Autodesk Inventor part; units mm, degrees
ref_plane "YZ Plane" through (0, 0, 0) normal (1, 0, 0) x (0, 1, 0)
ref_plane "XZ Plane" through (0, 0, 0) normal (0, 1, 0) x (-1, 0, 0)
ref_plane "XY Plane" through (0, 0, 0) normal (0, 0, 1) x (1, 0, 0)
sketch "Sketch1" plane through (0, 0, 0) normal (0, 0, 1) x (1, 0, 0)
  line L0 (-8.7146, 7.551) -> (3.2854, 7.551)
  line L1 (3.2854, 7.551) -> (3.2854, 3.051)
  line L2 (3.2854, 3.051) -> (-8.7146, 3.051)
  line L3 (-8.7146, 3.051) -> (-8.7146, 7.551)
  line L4 (2.7854, 7.051) -> (-8.2146, 7.051)
  line L5 (-8.2146, 7.051) -> (-8.2146, 3.551)
  line L6 (-8.2146, 3.551) -> (2.7854, 3.551)
  line L7 (2.7854, 3.551) -> (2.7854, 7.051)
  point P0 (0, 0)
  dimension "d0" = 12
  dimension "d1" = 4.5
  dimension "d2" = 0.5
extrude "Extrusion1" add sketch "Sketch1" along normal blind 15
properties part number "capa" material "Steel, Alloy"
CAD build for the part. Positions are in the model's coordinates, mm. A direction names the side the tool comes from. Round coordinates to 2 decimals unless told otherwise and drop trailing zeros. Write each loop counter-clockwise with the first axis right and the second up, starting at its lowest first coordinate (ties: lowest second). Pieces come first, ordered by that corner, then holes. Notation, with made-up numbers: (4, 28) - (52, 28) arc R32 ccw to (52, 65) - close; hole circle Ø5 at (7.25, -40). An arc over 180 degrees is marked (long way). Write item = value, one per line. Start each with the question number.
Q1. Probe L1, parallel to X at y = 5.65, z = 4.25; L2, parallel to Y at x = -1.5, z = 8.25. List the from-to ranges inside material, lowest first. Write a range as from..to.
Q2. Drop a flat-ended pin along its axis: pin 1 (2 mm diameter, centred on x = -3, y = 5, fed in from -Z). Give the stop position or say it passes through.
Q3. Band-saw the part on B-B (x = -5). Give the cut face in (y, z), then the cut area to 3 significant figures.
Q4. Band-saw the part on C-C (z = 9.25). Give the cut face in (x, y).
Q5. Which spindle directions (+Z, -Z, +X, -X, +Y, -Y) get a long thin tool onto all of the face, cutting with end or side? Do faces 5 (the flat face through (-3, 3.551, 7)), 6 (the flat face through (-3, 7.551, 7)). Say none if no direction does.
Q6. Mould opens along X. For faces 1 (the flat face through (-3, 7.051, 7)), 2 (the flat face through (-8.715, 5, 7)), 3 (the flat face through (-8.215, 5, 7)), 4 (the flat face through (-2.7, 3.3, 15)) say: pulls with the +X half, pulls with the -X half, needs draft (parallel to the pull), parting line crosses it, or undercut.
Q7. Band-saw the part on A-A (y = 5.8). Give the cut face in (x, z).
Answers below:
q1.L1 = -8.71..-8.21, 2.79..3.29
q1.L2 = 3.05..3.55, 7.05..7.55
q2.pin_1 = through
q3.outline = (3.05, 0) - (3.55, 0) - (3.55, 15) - (3.05, 15) - close; (7.05, 0) - (7.55, 0) - (7.55, 15) - (7.05, 15) - close
q3.area = 15.0 mm2
q4.outline = (-8.71, 3.05) - (3.29, 3.05) - (3.29, 7.55) - (-8.71, 7.55) - close; hole (-8.21, 3.55) - (2.79, 3.55) - (2.79, 7.05) - (-8.21, 7.05) - close
q5.face_5 = +Z, -Z
q5.face_6 = +Z, -Z, +X, -X, +Y
q6.face_1 = undercut
q6.face_2 = pulls with the -X half
q6.face_3 = undercut
q6.face_4 = needs draft
q7.outline = (-8.71, 0) - (-8.21, 0) - (-8.21, 15) - (-8.71, 15) - close; (2.79, 0) - (3.29, 0) - (3.29, 15) - (2.79, 15) - close
